Autodesk Inventor part; units mm, degrees
ref_plane "YZ Plane" through (0, 0, 0) normal (1, 0, 0) x (0, 1, 0)
ref_plane "XZ Plane" through (0, 0, 0) normal (0, 1, 0) x (-1, 0, 0)
ref_plane "XY Plane" through (0, 0, 0) normal (0, 0, 1) x (1, 0, 0)
sketch "Sketch1" plane through (0, 0, 0) normal (0, 1, 0) x (-1, 0, 0)
  line L0 (-50.8, 63.5) -> (50.8, 63.5)
  line L1 (50.8, 63.5) -> (50.8, -63.5)
  line L2 (50.8, -63.5) -> (-50.8, -63.5)
  line L3 (-50.8, -63.5) -> (-50.8, 63.5)
  line L4 (-50.8, 63.5) -> (50.8, -63.5) construction
  line L5 (50.8, 63.5) -> (-50.8, -63.5) construction
  point P0 (0, 0)
  dimension "d0" = 101.6
  dimension "d1" = 127
extrude "Extrusion1" add sketch "Sketch1" along normal blind 1.016
sketch "Sketch2" plane through (0, 1.016, 0) normal (0, 1, 0) x (1, 0, 0)
  line L0 (50.8, 63.5) -> (-50.8, 63.5)
  line L1 (50.8, -63.5) -> (-50.8, -63.5)
  line L2 (-50.8, -63.5) -> (-50.8, 63.5)
  line L3 (-50.8, 63.5) -> (50.8, 63.5)
  line L4 (50.8, 63.5) -> (50.8, -63.5)
  line L5 (50.8, -63.5) -> (-50.8, 63.5) construction
  line L6 (-50.8, -63.5) -> (50.8, 63.5) construction
  line L7 (50.292, -62.992) -> (-50.292, -62.992)
  line L8 (-50.292, -62.992) -> (-50.292, 62.992)
  line L9 (-50.292, 62.992) -> (50.292, 62.992)
  line L10 (50.292, 62.992) -> (50.292, -62.992)
  line L11 (50.292, -62.992) -> (-50.292, 62.992) construction
  line L12 (-50.292, -62.992) -> (50.292, 62.992) construction
  point P0 (0, 0)
  dimension "d4" = 100.584
  dimension "d5" = 125.984
extrude "Extrusion2" add sketch "Sketch2" along normal blind 76.2
sketch "Sketch3" plane through (0, 1.016, 0) normal (0, 1, 0) x (1, 0, 0)
  line L0 (0, 0) -> (0, -25.4)
  line L1 (0, -25.4) -> (0, 25.4)
  circle A0 centre (0, -25.4) radius 2.0828
  circle A1 centre (0, 25.4) radius 2.0828
  dimension "d8" = 25.4
  dimension "d9" = 50.8
  dimension "d10" = 4.1656
  dimension "d11" = 4.1656
extrude "Extrusion3" cut sketch "Sketch3" against normal through all
sketch "Sketch4" plane through (0, 1.016, 0) normal (0, 1, 0) x (1, 0, 0)
  line L0 (24.4983, -44.5008) -> (-24.4983, -44.5008)
  line L1 (-24.4983, 44.5008) -> (24.4983, 44.5008)
  line L2 (24.4983, 44.5008) -> (24.4983, -44.5008)
  line L3 (24.4983, -44.5008) -> (-24.4983, 44.5008) construction
  line L4 (-24.4983, -44.5008) -> (24.4983, 44.5008) construction
  line L5 (21.8694, -44.5008) -> (-21.8694, -44.5008)
  line L6 (-21.8694, 44.5008) -> (21.8694, 44.5008)
  line L7 (21.8694, -44.5008) -> (-21.8694, 44.5008) construction
  line L8 (-21.8694, -44.5008) -> (21.8694, 44.5008) construction
  line L9 (24.4983, 44.5008) -> (-24.4983, 44.5008)
  line L10 (-24.4983, 44.5008) -> (-24.4983, -24.511)
  line L11 (24.4983, -24.511) -> (24.4983, 44.5008)
  line L12 (-21.8694, -44.5008) -> (-18.6944, -44.5008)
  line L13 (21.8694, -44.5008) -> (18.6944, -44.5008)
  line L14 (24.4983, 44.5008) -> (21.3233, 44.5008)
  line L15 (24.4983, 41.3258) -> (24.4983, 44.5008)
  line L16 (-24.4983, 44.5008) -> (-21.3233, 44.5008)
  line L17 (-24.4983, 41.3258) -> (-24.4983, 44.5008)
  circle A0 centre (-18.6944, -41.3258) radius 1.4224
  circle A1 centre (-21.3233, 41.3258) radius 1.4224
  circle A2 centre (21.3233, 41.3258) radius 1.4224
  circle A3 centre (18.6944, -41.3258) radius 1.4224
  point P0 (0, 0)
  dimension "d14" = 48.9966
  dimension "d15" = 89.0016
  dimension "d16" = 43.7388
  dimension "d17" = 89.0016
  dimension "d18" = 69.0118
  dimension "d27" = 2.8448
  dimension "d28" = 2.8448
  dimension "d29" = 2.8448
  dimension "d30" = 2.8448
extrude "Extrusion4" cut sketch "Sketch4" against normal through all
sketch "Sketch5" plane through (0, 1.016, 0) normal (0, 1, 0) x (1, 0, 0)
  line L0 (9.9949, -32.9946) -> (-9.9949, -32.9946)
  line L1 (-9.9949, 32.9946) -> (9.9949, 32.9946)
  line L2 (9.9949, 32.9946) -> (9.9949, -32.9946)
  line L3 (9.9949, -32.9946) -> (-9.9949, 32.9946) construction
  line L4 (-9.9949, -32.9946) -> (9.9949, 32.9946) construction
  circle A0 centre (-9.9949, -32.9946) radius 1.4224
  circle A1 centre (9.9949, -32.9946) radius 1.4224
  circle A2 centre (9.9949, 32.9946) radius 1.4224
  circle A3 centre (-9.9949, 32.9946) radius 1.4224
  point P0 (0, 0)
  dimension "d33" = 19.9898
  dimension "d34" = 65.9892
  dimension "d35" = 2.8448
  dimension "d36" = 2.8448
  dimension "d37" = 2.8448
  dimension "d38" = 2.8448
extrude "Extrusion5" cut sketch "Sketch5" against normal through all
sketch "Sketch6" plane through (-50.292, 1.016, 62.992) normal (1, 0, 0) x (0, 0, -1)
  line L0 (0, 0) -> (0, 76.2)
  line L1 (0, 19.05) -> (18.4912, 19.05)
  line L2 (0, 19.05) -> (18.4912, 19.05) construction
  line L3 (18.4912, 19.05) -> (29.6164, 19.05)
  line L4 (29.6164, 19.05) -> (58.1914, 19.05)
  circle A0 centre (29.6164, 19.05) radius 3.175
  circle A1 centre (58.1914, 19.05) radius 3.175
  point P0 (62.992, -1.016)
  dimension "d41" = 18.4912
  dimension "d42" = 0
  dimension "d43" = 11.1252
  dimension "d44" = 28.575
  dimension "d45" = 180
  dimension "d46" = 6.35
  dimension "d47" = 6.35
extrude "Extrusion6" cut sketch "Sketch6" against normal through all
sketch "Sketch7" plane through (50.292, 1.016, -62.992) normal (-1, 0, 0) x (0, 0, 1)
  line L0 (125.984, 0) -> (125.984, 76.2)
  line L1 (125.984, 19.05) -> (107.4928, 19.05)
  line L2 (125.984, 19.05) -> (144.4752, 19.05) construction
  line L3 (107.4928, 19.05) -> (96.3676, 19.05)
  line L4 (96.3676, 19.05) -> (67.7926, 19.05)
  circle A0 centre (67.7926, 19.05) radius 3.175
  circle A1 centre (96.3676, 19.05) radius 3.175
  point P0 (62.992, -1.016)
  dimension "d50" = 18.4912
  dimension "d51" = 180
  dimension "d52" = 11.1252
  dimension "d53" = 28.575
  dimension "d54" = 180
  dimension "d55" = 6.35
  dimension "d56" = 6.35
extrude "Extrusion7" cut sketch "Sketch7" against normal through all
properties part number "563-AU1028MG-PE4312"
The listing builds one solid part. Answer for the finished solid, in the listing's coordinates (mm). A direction names the side the tool comes from. Give positions to 0.01 mm unless a question says otherwise; leave off trailing zeros. Write each loop counter-clockwise with the first axis right and the second up, starting at its lowest first coordinate (ties: lowest second). Pieces come first, ordered by that corner, then holes. Notation, with made-up numbers: (47, 66) - (102, 66) arc R18 ccw to (102, 96) - close; hole circle Ø11 at (85.5, 4). An arc over 180 degrees is marked (long way). Use one line per item in the form item = value. Start each with the question number.
1) A tool of negligible diameter and unlimited length cuts with its end or side. For faces 4 (the face through (-50.542, 23.214, 5.214)), 5 (the face through (50.292, 39, -1)), from which of +Z, -Z, +X, -X, +Y, -Y can it reach the whole face along a straight path? Write none if from no direction.
2) Find section A-A on x = 0. Determine the outline of the cut face in (y, z), plus the area to 3 significant figures.
3) Find section C-C on z = 25.4. Determine the outline of the cut face in (x, y), plus the area to 3 significant figures.
4) Find section D-D on x = -27. Determine the outline of the cut face in (y, z).
5) Find section B-B on y = 44.5. Determine the outline of the cut face in (x, z), plus the area to 3 significant figures.
6) The mould has two halves that part along X. Classify faces 1 (the face through (-1, 38, -63.5)), 2 (the face through (-1, 39, -62.992)), 3 (the face through (50.8, 38, -1)): pulls with the +X half, pulls with the -X half, needs draft (parallel to the pull), parting line crosses it, or undercut.
7) A flat-ended cylindrical pin translates along its axis: pin 1 Ø6 at (x, z) = (38.5, -7.5) entering from +Y. Find the tip coordinate at first contact, or state that the pin passes through.
8) Consider line 1 along Z through (x, y) = (0, 0.35); line 2 along X through (y, z) = (58.5, 12); line 3 along Z through (x, y) = (-42.5, 47). Determine where each line is inside the solid, lowest interval first. Write a range as from..to.
Geometry results:
q1.face_4 = +X, -X
q1.face_5 = +Y
q2.outline = (0, -63.5) - (77.22, -63.5) - (77.22, -62.99) - (1.02, -62.99) - (1.02, -27.48) - (0, -27.48) - close; (0, -23.32) - (1.02, -23.32) - (1.02, 23.32) - (0, 23.32) - close; (0, 27.48) - (1.02, 27.48) - (1.02, 62.99) - (77.22, 62.99) - (77.22, 63.5) - (0, 63.5) - close
q2.area = 198 mm2
q3.outline = (-50.8, 0) - (-2.08, 0) - (-2.08, 1.02) - (-50.29, 1.02) - (-50.29, 77.22) - (-50.8, 77.22) - close; (2.08, 0) - (50.8, 0) - (50.8, 77.22) - (50.29, 77.22) - (50.29, 1.02) - (2.08, 1.02) - close
q3.area = 176 mm2
q4.outline = (0, -63.5) - (77.22, -63.5) - (77.22, -62.99) - (1.02, -62.99) - (1.02, 62.99) - (77.22, 62.99) - (77.22, 63.5) - (0, 63.5) - close
q5.outline = (-50.8, -63.5) - (50.8, -63.5) - (50.8, 63.5) - (-50.8, 63.5) - close; hole (-50.29, -62.99) - (50.29, -62.99) - (50.29, 62.99) - (-50.29, 62.99) - close
q5.area = 231 mm2
q6.face_1 = needs draft
q6.face_2 = undercut
q6.face_3 = pulls with the +X half
q7.pin_1 = 1.02
q8.line_1 = -63.5..-27.48, -23.32..23.32, 27.48..63.5
q8.line_2 = -50.8..-50.29, 50.29..50.8
q8.line_3 = -63.5..-62.99, 62.99..63.5
